Verification items for the finished model (mm, model axes). A direction names the side the tool comes from. Round coordinates to 2 decimals unless told otherwise and drop trailing zeros. Order: outer loops, then holes, each group sorted by start corner. A loop starts at its lowest first (then second) coordinate and runs counter-clockwise, first axis right, second up. Notation, with made-up numbers: M -31,75.25 L -18,75.25 A24 cw -18,112.25 Z; hole C 32.25,-1.75 d2. An arc over 180 degrees is marked long. Use CSV: the item, a comma, the result in double quotes. Start each with the question number.
Q1. Mould release check, pull along Z, two halves, no side actions. Record for faces 4 (the face through (40, 3, -6.5)), 5 (the face through (82.487, 1.972, -0.195)), 6 (the face through (99.873, 2.958, 32.403)): +Z half, -Z half, draft (parallel to the pull), parting line (faces both ways), or undercut.
Q2. Sectioned sample at A-A (z = 0). Enter the section's corners in (x, y).
Q3. Scan lines: line 1 (Z direction, x = 81, y = 2.3); line 2 (Z direction, x = 0, y = 2.2); line 3 (X direction, y = 4.9, z = 0). Record each from-to range of solid material in increasing order.
Q4. Gauge pin test, flat ends, axial feed: pin 1 Ø1 at (y, z) = (2.5, 5) entering from -X; pin 2 Ø2.5 at (x, z) = (96.5, 26.85) entering from +Y; pin 3 Ø4.5 at (x, z) = (-1.5, 1.5) entering from +Y; pin 4 Ø7 at (x, z) = (79.5, 0) entering from +Y. Record the tip position at first contact, or that the pin passes through.
Q5. Sectioned sample at B-B (x = 96.5). Enter the section's corners in (y, z), and give its area (3 significant figures).
Q6. Sectioned sample at D-D (y = 8). Enter the section's corners in (x, z) (3 decimals).
Q7. Sectioned sample at C-C (y = 1.5). Enter the section's corners in (x, z).
Q8. Set-up check for faces 1 (the face through (-2, 4, 0)), 2 (the face through (36, 3, 6.5)), 3 (the face through (-6.5, 3, 0.1)): record each of +Z, -Z, +X, -X, +Y, -Y from which the full face is reachable in a straight line by a thin tool's end or side.
```python
from build123d import *

# Parameters (mm, degrees)
SKETCH1_R           = 1.5
BOSS_EXTRUDE1_DEPTH = 6
SKETCH2_R           = 4.5
CUT_EXTRUDE1_DEPTH  = 2
SKETCH3_R           = 3.975
SKETCH3_R_2         = 1.5
BOSS_EXTRUDE2_DEPTH = 7


with BuildPart() as part:
    # Sketch1 → Boss-Extrude1 (new body)
    with BuildSketch(Plane(origin=(0, 0, 0), x_dir=(1, 0, 0), z_dir=(0, 1, 0))):
        with BuildLine():
            Line((0, 6.5), (81, 6.5))
            ThreePointArc((81, 6.5), (84.25, 5.629165125), (86.629165125, 3.25))
            Line((86.629165125, 3.25), (102.129165125, -23.596787517))
            ThreePointArc((102.129165125, -23.596787517), (99.75, -32.475952642), (90.870834875, -30.096787517))
            Line((90.870834875, -30.096787517), (80.133974596, -11.5))
            ThreePointArc((80.133974596, -11.5), (76.473720558, -7.839745962), (71.473720558, -6.5))
            Line((71.473720558, -6.5), (0, -6.5))
            ThreePointArc((0, -6.5), (-6.5, 0), (0, 6.5))
        make_face()
        with Locations(Location((0, 0, 0), (0, 0, 270))):
            Circle(SKETCH1_R, mode=Mode.SUBTRACT)
        with Locations(Location((81, 0, 0), (0, 0, 270))):
            Circle(SKETCH1_R, mode=Mode.SUBTRACT)
        with Locations(Location((96.5, -26.846787517, 0), (0, 0, 270))):
            Circle(SKETCH1_R, mode=Mode.SUBTRACT)
    extrude(amount=BOSS_EXTRUDE1_DEPTH)

    # Sketch2 → Cut-Extrude1 (cut)
    with BuildSketch(Plane(origin=(0, 6, 0), x_dir=(1, 0, 0), z_dir=(0, 1, 0))):
        with Locations(Location((0, 0, 0), (0, 0, 270))):
            Circle(SKETCH2_R)
        with Locations(Location((81, 0, 0), (0, 0, 270))):
            Circle(SKETCH2_R)
    extrude(amount=-CUT_EXTRUDE1_DEPTH, mode=Mode.SUBTRACT)

    # Sketch3 → Boss-Extrude2 (add)
    with BuildSketch(Plane(origin=(0, 6, 0), x_dir=(1, 0, 0), z_dir=(0, 1, 0))):
        with Locations(Location((96.5, -26.846787517, 0), (0, 0, 270))):
            Circle(SKETCH3_R)
        with Locations(Location((96.5, -26.846787517, 0), (0, 0, 270))):
            Circle(SKETCH3_R_2, mode=Mode.SUBTRACT)
    extrude(amount=BOSS_EXTRUDE2_DEPTH)


solid = part.part
```
Verdict:
1,face 4,"-Z half"
1,face 5,"undercut"
1,face 6,"parting line"
2,outline,"M -6.5,0 L -1.5,0 L -1.5,4 L -4.5,4 L -4.5,6 L -6.5,6 Z; M 1.5,0 L 79.5,0 L 79.5,4 L 76.5,4 L 76.5,6 L 4.5,6 L 4.5,4 L 1.5,4 Z; M 82.5,0 L 88.51,0 L 88.51,6 L 85.5,6 L 85.5,4 L 82.5,4 Z"
3,line 1,"z = -6.5 to -1.5, 1.5 to 13"
3,line 2,"z = -6.5 to -1.5, 1.5 to 6.5"
3,line 3,"x = -6.5 to -4.5, 4.5 to 76.5, 85.5 to 88.51"
4,pin 1,"stops at x = -4.69"
4,pin 2,"passes through"
4,pin 3,"stops at y = 4"
4,pin 4,"stops at y = 6"
5,outline,"M 0,13.85 L 6,13.85 L 6,22.87 L 13,22.87 L 13,25.35 L 0,25.35 Z; M 0,28.35 L 13,28.35 L 13,30.82 L 6,30.82 L 6,33.35 L 0,33.35 Z"
5,area,"134 mm²"
6,outline,"C 96.5,26.847 d7.95; hole C 96.5,26.847 d3"
7,outline,"M 0,-6.5 L 81,-6.5 A6.5 ccw 86.63,-3.25 L 102.13,23.6 A6.5 ccw 90.87,30.1 L 80.13,11.5 A10 cw 71.47,6.5 L 0,6.5 A6.5 ccw Z; hole C 0,0 d3; hole C 81,0 d3; hole C 96.5,26.85 d3"
8,face 1,"+Y"
8,face 2,"+Z, -X, +Y, -Y"
8,face 3,"-X, +Y, -Y"
